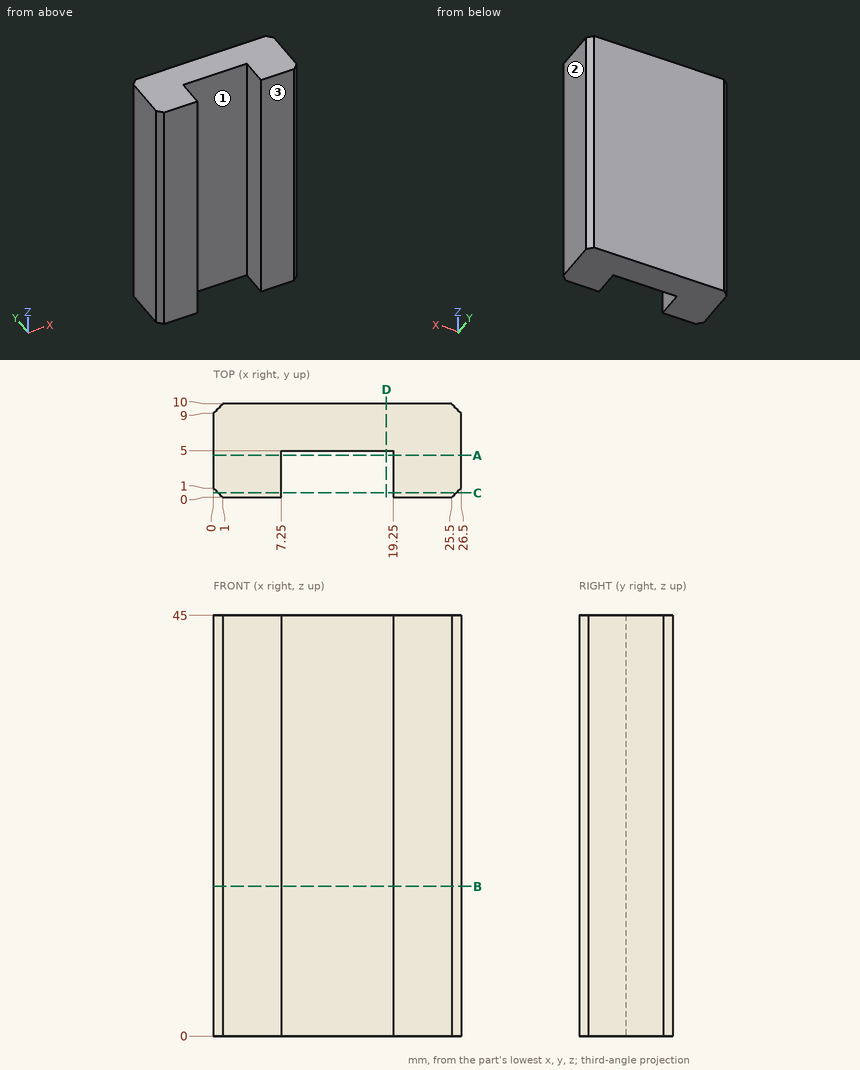
For this review, use the dimensioned drawing (mm, ordinates from the lowest corner) and the shaded views. Give positions to 0.01 mm unless a question says otherwise; leave off trailing zeros. Write each loop counter-clockwise with the first axis right and the second up, starting at its lowest first coordinate (ties: lowest second). Pieces come first, ordered by that corner, then holes.
(1) Consider section D-D, the plane x = 18.5. Give the boundary of the cut face in (y, z).
(2) For P1, Ø6, axis at x = 10.5, z = 23.5, coming from the -Y side, flat-tipped, find the tip position at first contact; note if it passes through.
(3) Consider section C-C, the plane y = 0.5. Give the boundary of the cut face in (x, z).
(4) Consider section B-B, the plane z = 16. Give the boundary of the cut face in (x, y), and give its area (3 significant figures).
(5) To check wall thickness, follow L1, parallel to X at y = 4.5, z = 37; L2, parallel to Y at x = 15.25, z = 13. State the ranges of each line that lie inside material, in increasing order.
(6) Consider section A-A, the plane y = 4.5. Give the boundary of the cut face in (x, z).
(7) The part is to be moulded in two halves that separate along X. For the marked faces 1, 2 and 3, say which applies: released by +X, released by -X, zero draft, split by the parting line, or undercut.
Returned:
1. outline: (5, 0) - (10, 0) - (10, 45) - (5, 45) - close
2. P1: stops at y = 5
3. outline: (0.5, 0) - (7.25, 0) - (7.25, 45) - (0.5, 45) - close; (19.25, 0) - (26, 0) - (26, 45) - (19.25, 45) - close
4. outline: (0, 1) - (1, 0) - (7.25, 0) - (7.25, 5) - (19.25, 5) - (19.25, 0) - (25.5, 0) - (26.5, 1) - (26.5, 9) - (25.5, 10) - (1, 10) - (0, 9) - close
4. area: 203 mm2
5. L1: x = 0 to 7.25, 19.25 to 26.5
5. L2: y = 5 to 10
6. outline: (0, 0) - (7.25, 0) - (7.25, 45) - (0, 45) - close; (19.25, 0) - (26.5, 0) - (26.5, 45) - (19.25, 45) - close
7. face 1: undercut
7. face 2: released by +X
7. face 3: zero draft
